For this review, use the dimensioned drawing (mm, ordinates from the lowest corner) and the shaded views. Round coordinates to 2 decimals unless told otherwise and drop trailing zeros. Loops run counter-clockwise (first coordinate to the right, second up) from the corner with the lowest first, then second, coordinate; pieces in that order, holes last. Notation, with made-up numbers: (7, 18.5) - (52, 18.5) arc R18 cw to (52, 22.5) - close; hole circle Ø2 at (52, 12.5). An arc over 180 degrees is marked (long way). Use one line per item in the form item = value. Start each with the question number.
(1) We need section A-A, the plane x = 17.7. Write out the cut boundary in (y, z).
(2) We need section C-C, the plane x = 50.7. Write out the cut boundary in (y, z), then the cut area to 3 significant figures.
(3) For pin 1 (2 mm diameter, centred on x = 50.7, z = 88.9, fed in from +Y); pin 2 (4 mm diameter, centred on x = 50.7, z = 6.55, fed in from -Y), all flat-tipped, find the tip position at first contact; note any pin that passes through.
(4) Wall thickness on probe 1 along Z at (x, y) = (2.5, 2.75); probe 2 along X at (y, z) = (1.5, 36.8); probe 3 along Z at (x, y) = (50.7, 3.5): over which ranges is each line inside the solid? List them lowest first. Write a range as [from, to].
(5) We need section D-D, the plane z = 36.8. Write out the cut boundary in (x, y).
(6) We need section B-B, the plane z = 6.55. Write out the cut boundary in (x, y), then the cut area to 3 significant figures.
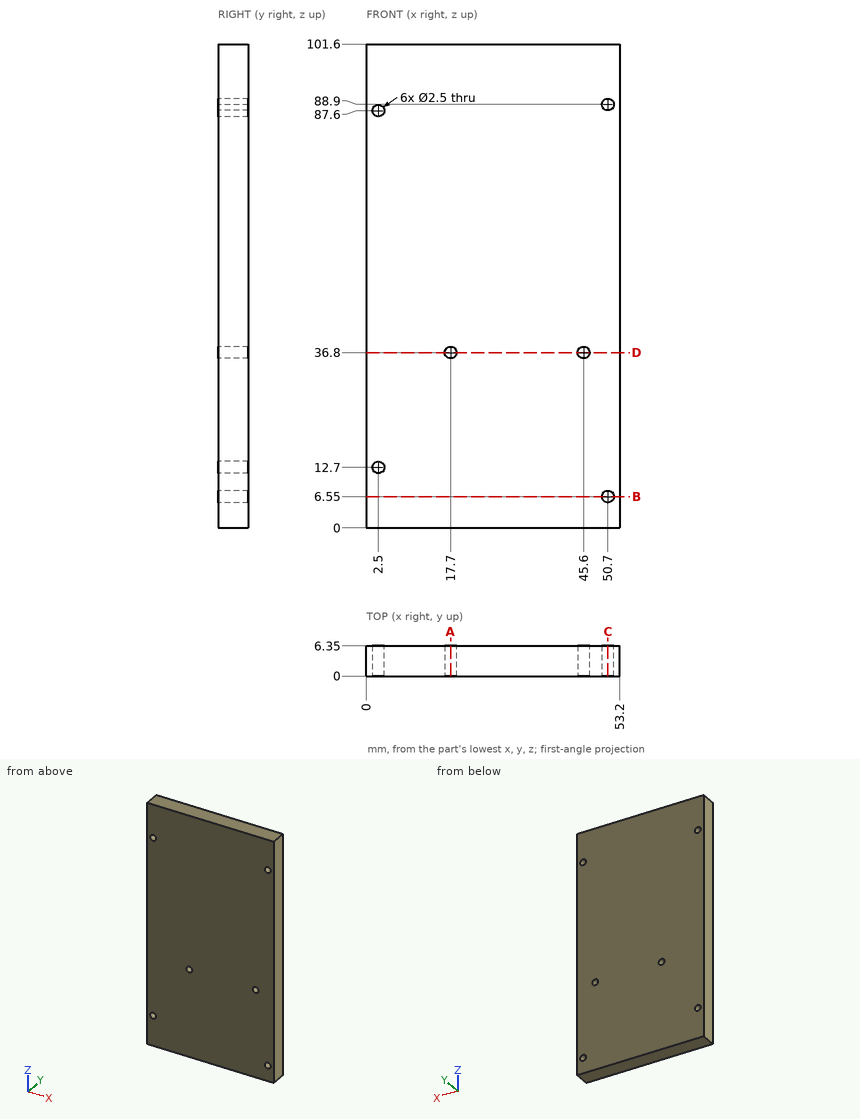
Data:
q1.outline = (0, 0) - (6.35, 0) - (6.35, 35.55) - (0, 35.55) - close; (0, 38.05) - (6.35, 38.05) - (6.35, 101.6) - (0, 101.6) - close
q2.outline = (0, 0) - (6.35, 0) - (6.35, 5.3) - (0, 5.3) - close; (0, 7.8) - (6.35, 7.8) - (6.35, 87.65) - (0, 87.65) - close; (0, 90.15) - (6.35, 90.15) - (6.35, 101.6) - (0, 101.6) - close
q2.area = 613 mm^2
q3.pin_1 = through
q3.pin_2 = 0
q4.probe_1 = [0, 11.45], [13.95, 86.35], [88.85, 101.6]
q4.probe_2 = [0, 16.45], [18.95, 44.35], [46.85, 53.2]
q4.probe_3 = [0, 5.3], [7.8, 87.65], [90.15, 101.6]
q5.outline = (0, 0) - (16.45, 0) - (16.45, 6.35) - (0, 6.35) - close; (18.95, 0) - (44.35, 0) - (44.35, 6.35) - (18.95, 6.35) - close; (46.85, 0) - (53.2, 0) - (53.2, 6.35) - (46.85, 6.35) - close
q6.outline = (0, 0) - (49.45, 0) - (49.45, 6.35) - (0, 6.35) - close; (51.95, 0) - (53.2, 0) - (53.2, 6.35) - (51.95, 6.35) - close
q6.area = 322 mm^2
